Build history of the part. All positions in model axes, mm. A direction names the side the tool comes from. Give positions to 0.01 mm unless a question says otherwise; leave off trailing zeros. Loops run counter-clockwise (first coordinate to the right, second up) from the corner with the lowest first, then second, coordinate; pieces in that order, holes last. Notation, with made-up numbers: (-7, 25) -> (8, 25) arc R17 cw to (8, 44) -> close; hole circle Ø2 at (-2.5, 50.25). An arc over 180 degrees is marked (long way). Answer as a JSON object with one key per item and string values. Group by question number.
Q1. Tool access for faces 4 (the conical face through (-15.8, 0, -15.6)), 5 (the flat face through (-11, -14, 1)), 6 (the cylindrical face through (-11.306, 12.056, -3.301)): list every direction of +Z, -Z, +X, -X, +Y, -Y with a clear straight run to the whole face (end or side of a thin tool).
Q2. Band-saw the part on C-C, the plane z = 0. Write the cut outline in (x, y), plus the area to 3 significant figures.
Q3. Drop flat-ended pins along their axis: pin 1 (6 mm diameter, centred on y = 16.865, z = 0, fed in from -X); pin 2 (3 mm diameter, centred on y = 0, z = -16.865, fed in from +X); pin 3 (1 mm diameter, centred on x = -14.5, y = 13, fed in from -Z); pin 4 (4 mm diameter, centred on x = -7, y = -14, fed in from +Z). Give the stop position or say it passes through.
Q4. Band-saw the part on A-A, the plane y = 0. Write the cut outline in (x, z), plus the area to 3 significant figures.
Q5. Two-plate mould, pull along Z, no slides. Class faces 1 (the cylindrical face through (-7.61, 14.27, -0.06)), 2 (the conical face through (-15.8, 0, 15.6)), 3 (the flat face through (0, 5, 12)): pulls with the +Z half, pulls with the -Z half, needs draft (parallel to the pull), parting line crosses it, or undercut.
Q6. Band-saw the part on D-D, the plane x = -18.75. Write the cut outline in (y, z).
Q7. Wall check: probe 1 along Z at (x, y) = (-6.25, 0); probe 2 along Y at (x, z) = (-10, 0); probe 3 along Z at (x, y) = (-11.5, -6). Give the ranges that are in metal, low to high. Write a range as from..to.
Autodesk Inventor part; units mm, degrees
ref_plane "YZ Plane" through (0, 0, 0) normal (1, 0, 0) x (0, 1, 0)
ref_plane "XZ Plane" through (0, 0, 0) normal (0, 1, 0) x (-1, 0, 0)
sketch "Esquisse1" plane through (0, 0, 0) normal (0, 0, 1) x (1, 0, 0)
  line L0 (-36.1898, 0) -> (37.2521, 0)
  line L1 (0, 12.5) -> (-22.3, 12.5)
  line L2 (-22.3, 12.5) -> (-22.3, 16)
  line L3 (-22.3, 16) -> (0, 17.6)
  line L4 (0, 17.6) -> (0, 12.5)
  point P0 (0, 0)
  dimension "d0" = 25
  dimension "d1" = 35.2
  dimension "d2" = 0
  dimension "d3" = 32
  dimension "d4" = 22.3
  dimension "d5" = 0
revolve "Révolution1" add sketch "Esquisse1" angle 360 about axis through (-36.1898, 0, 0) along (1, 0, 0)
sketch "Esquisse4" plane through (0, 0, 0) normal (1, 0, 0) x (0, 0, 1)
  line L0 (0, 0) -> (-39.036, -39.036)
  line L1 (0, 0) -> (-55.3193, 0)
  circle A0 centre (0, 0) radius 12.5
  line L2 (-5.5456, -11.2025) -> (-6.4649, -12.1217)
  line L3 (-11.2025, -5.5456) -> (-12.1217, -6.4649)
  line L4 (-12.1217, -6.4649) -> (-6.4649, -12.1217)
  dimension "d17" = 45
  dimension "d20" = 1.3
  dimension "d21" = 1.3
  dimension "d22" = 4
  dimension "d23" = 4
extrude "Extrusion1" cut sketch "Esquisse4" against normal through all contours A0 L2 L4 L0 | L0 L4 L3 A0
sketch "Esquisse5" plane through (0, 0, 0) normal (1, 0, 0) x (0, 0, 1)
  line L0 (-1, 17.6) -> (1, 17.6)
  line L1 (1, 17.6) -> (1, -13.4)
  line L2 (1, -13.4) -> (-1, -13.4)
  line L3 (-1, -13.4) -> (-1, 17.6)
  line L4 (-1, 17.6) -> (1, -13.4) construction
  line L5 (1, 17.6) -> (-1, -13.4) construction
  arc A0 (0, -17.6) -> (0, -17.6) centre (0, 0) ccw
  point P0 (0, 2.1)
  dimension "d26" = 2
  dimension "d27" = 31
  dimension "d28" = 0
extrude "Extrusion2" cut sketch "Esquisse5" against normal through all contours L0 A0 L3 | L0 L1 A0 | A0 L1 L2 L3 picked at (0, -3.0667)
sketch "Esquisse6" plane through (0, 0, 0) normal (1, 0, 0) x (0, 0, -1)
  line L0 (0, 0) -> (0, 23.579)
  line L1 (0, 0) -> (-21.6871, 0)
  line L2 (0, 0) -> (25.1017, 0)
  circle A0 centre (0, 0) radius 16.865
  point P0 (0, 16.865)
  point P1 (16.865, 0)
  point P2 (-16.865, 0)
  dimension "d39" = 33.73
hole "Perçage2" at (0, 16.865, 0) at (0, 0, -16.865) at (0, 0, 16.865) direction (-1, 0, 0) diameter 5.1881 depth 15 tip angle 118
properties part number "Douille1008"
Worked answers:
{
 "1": {"face 4": "-Z, +X", "face 5": "+X, -X, -Y", "face 6": "+X, -X"},
 "2": {"outline": "(-22.3, 13.4) -> (0, 13.4) -> (0, 14.27) -> (-15, 14.27) -> (-16.3, 16.43) -> (-22.3, 16) -> close", "area": "32.5 mm2"},
 "3": {"pin 1": "x = -22.3", "pin 2": "x = -15.66", "pin 3": "z = -10.86", "pin 4": "z = 12.19"},
 "4": {"outline": "(-22.3, -16) -> (-16.3, -16.43) -> (-15, -14.27) -> (0, -14.27) -> (0, -12.5) -> (-22.3, -12.5) -> close; (-22.3, 12.5) -> (0, 12.5) -> (0, 14.27) -> (-15, 14.27) -> (-16.3, 16.43) -> (-22.3, 16) -> close", "area": "105 mm2"},
 "5": {"face 1": "undercut", "face 2": "pulls with the +Z half", "face 3": "needs draft"},
 "6": {"outline": "(-16.22, -1) arc R16.25 ccw (long way) to (-16.22, 1) -> (-12.46, 1) arc R12.5 cw to (12.46, 1) -> (13.4, 1) -> (13.4, -1) -> (12.46, -1) arc R12.5 cw to (11.2, -5.55) -> (12.12, -6.46) -> (6.46, -12.12) -> (5.55, -11.2) arc R12.5 cw to (-12.46, -1) -> close"},
 "7": {"probe 1": "-14.27..-12.5, 12.5..14.27", "probe 2": "13.4..14.27", "probe 3": "-15.67..-10.97, 10.97..15.67"}
}
